Design review of the part shown in the three views and the two pictorial views. Dimensions are in mm from the part's minimum x, y and z. Give positions to 0.01 mm unless a question says otherwise; leave off trailing zeros. Loops run counter-clockwise (first coordinate to the right, second up) from the corner with the lowest first, then second, coordinate; pieces in that order, holes last.
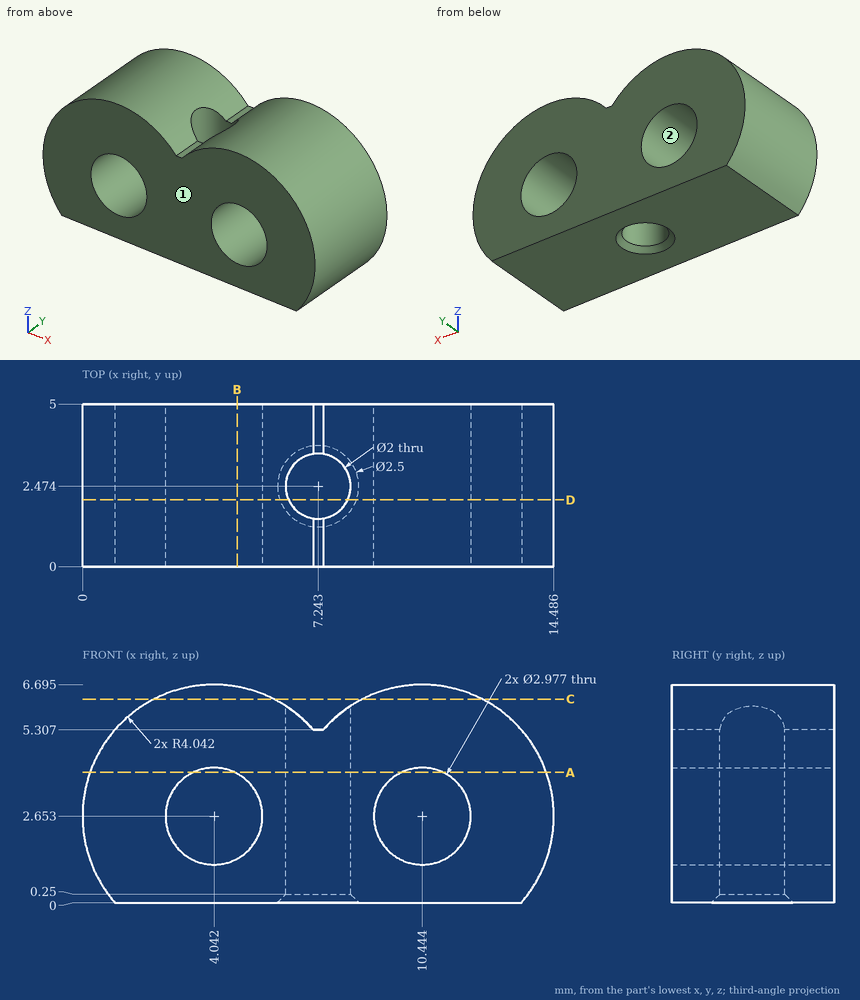
Q1. Consider section B-B on x = 4.75. Give the boundary of the cut face in (y, z).
Answers:
outline: (0, 0) - (5, 0) - (5, 1.34) - (0, 1.34) - close; (0, 3.96) - (5, 3.96) - (5, 6.63) - (0, 6.63) - close
Q2. Mouldability with a two-part tool opening along X and no side actions: class the marked faces 1 and 2 as +X half, -X half, draft (parallel to the pull), parting line (faces both ways), or undercut.
Answers:
face 1: draft
face 2: undercut
Q3. For pin 1 Ø1.5 at (x, y) = (5.5, 3.5) entering from +Z; pin 2 Ø2.5 at (x, y) = (7.24, 2.47) entering from +Z (1 decimal), all flat-tipped, find the tip position at first contact; note any pin that passes through.
Answers:
pin 1: stops at z = 6.63
pin 2: stops at z = 6.2
Q4. Consider section D-D on y = 2.05. Count the separate pieces of the cut face and the enclosed holes in it.
Answers:
separate pieces: 2
enclosed holes: 2
Q5. Consider section C-C on z = 6.25. Give the boundary of the cut face in (x, y).
Answers:
outline: (2.2, 0) - (5.89, 0) - (5.89, 5) - (2.2, 5) - close; (8.6, 0) - (12.29, 0) - (12.29, 5) - (8.6, 5) - close
Q6. For probe 1 along X at (y, z) = (0.4, 2) (1 decimal); probe 2 along X at (y, z) = (4.45, 3) (1 decimal); probe 3 along Z at (x, y) = (10, 1.9) (1 decimal), list the stretches that pass through material, from the lowest coordinate up.
Answers:
probe 1: x = 0.1 to 2.7, 5.4 to 9.1, 11.8 to 14.4
probe 2: x = 0 to 2.6, 5.5 to 9, 11.9 to 14.5
probe 3: z = 0 to 1.2, 4.1 to 6.7
Q7. Consider section A-A on z = 4. Give the boundary of the cut face in (x, y) (1 decimal).
Answers:
outline: (0.2, 0) - (3.4, 0) - (3.4, 5) - (0.2, 5) - close; (4.7, 0) - (9.8, 0) - (9.8, 5) - (4.7, 5) - close; (11.1, 0) - (14.3, 0) - (14.3, 5) - (11.1, 5) - close; hole circle Ø2 at (7.2, 2.5)
